Design review of the part built by this model. Coordinates are the model's own, in mm. Face numbers are marked on the shaded views. Give positions to 0.01 mm unless a question says otherwise; leave off trailing zeros. Order: outer loops, then holes, each group sorted by start corner. A loop starts at its lowest first (then second) coordinate and runs counter-clockwise, first axis right, second up. Notation, with made-up numbers: (59.5, 19.5) -> (86.5, 19.5) arc R27 ccw to (86.5, 36.5) -> close; hole circle Ø10 at (-19.5, 1). An arc over 180 degrees is marked (long way). Use a Markdown table: item, result. Add a question column.
```python
from build123d import *

# Parameters (mm, degrees)
BOSS_EXTRUDE1_DEPTH = 0.508
SKETCH2_R           = 7.874
SKETCH2_R_2         = 6.35
CUT_EXTRUDE2_DEPTH  = 0.254
SKETCH5_R           = 6.354160617
CUT_EXTRUDE3_DEPTH  = 68.821805137
SKETCH6_R           = 5.461
CUT_EXTRUDE4_DEPTH  = 68.821805137
SKETCH7_W           = 19.558
SKETCH7_H           = 1.016
CUT_EXTRUDE5_DEPTH  = 68.823232008
SKETCH8_W           = 6.35
SKETCH8_H           = 0.254
BOSS_EXTRUDE2_DEPTH = 2.032
SKETCH10_W          = 11.303182767
SKETCH10_H          = 0.254
BOSS_EXTRUDE3_DEPTH = 2.032
SKETCH11_W          = 6.35
SKETCH11_H          = 0.254
BOSS_EXTRUDE4_DEPTH = 2.032
SKETCH12_W          = 11.938
SKETCH12_H          = 0.254
BOSS_EXTRUDE5_DEPTH = 2.032


with BuildPart() as part:
    # Sketch1 → Boss-Extrude1 (new body)
    with BuildSketch(Plane.XY):
        with BuildLine():
            ThreePointArc((0, -10.16), (10.16, 0), (0, 10.16))
            Line((0, 10.16), (-67.056, 10.16))
            Line((-67.056, 10.16), (-67.056, -10.16))
            Line((-67.056, -10.16), (0, -10.16))
        make_face()
    extrude(amount=BOSS_EXTRUDE1_DEPTH)

    # Sketch2 → Cut-Extrude2 (cut)
    with BuildSketch(Plane.XY.offset(0.508)):
        with Locations((-54.61, 0)):
            Circle(SKETCH2_R)
        with Locations((-35.814, 0)):
            Circle(SKETCH2_R_2)
    extrude(amount=-CUT_EXTRUDE2_DEPTH, mode=Mode.SUBTRACT)

    # Sketch5 → Cut-Extrude3 (cut, through all)
    with BuildSketch(Plane.XY.offset(0.254)):
        with Locations((-35.814, 0)):
            Circle(SKETCH5_R)
    extrude(amount=-CUT_EXTRUDE3_DEPTH, mode=Mode.SUBTRACT)

    # Sketch6 → Cut-Extrude4 (cut, through all)
    with BuildSketch(Plane.XY.offset(0.254)):
        with Locations((-54.61, 0)):
            Circle(SKETCH6_R)
    extrude(amount=-CUT_EXTRUDE4_DEPTH, mode=Mode.SUBTRACT)

    # Sketch7 → Cut-Extrude5 (cut, through all)
    with BuildSketch(Plane(origin=(0, 0, 0), x_dir=(-1, 0, 0), z_dir=(0, 0, -1))):
        with Locations((50.927, 9.652)):
            Rectangle(SKETCH7_W, SKETCH7_H)
        with Locations((50.927, -9.652)):
            Rectangle(SKETCH7_W, SKETCH7_H)
    extrude(amount=-CUT_EXTRUDE5_DEPTH, mode=Mode.SUBTRACT)

    # Sketch8 → Boss-Extrude2 (add)
    with BuildSketch(Plane(origin=(0, 0, 0), x_dir=(-1, 0, 0), z_dir=(0, 0, -1))):
        with Locations((63.881, 10.033)):
            Rectangle(SKETCH8_W, SKETCH8_H)
    extrude(amount=BOSS_EXTRUDE2_DEPTH)

    # Sketch10 → Boss-Extrude3 (add)
    with BuildSketch(Plane(origin=(0, 0, 0), x_dir=(-1, 0, 0), z_dir=(0, 0, -1))):
        with Locations((35.496408617, 10.033)):
            Rectangle(SKETCH10_W, SKETCH10_H)
    extrude(amount=BOSS_EXTRUDE3_DEPTH)

    # Sketch11 → Boss-Extrude4 (add)
    with BuildSketch(Plane(origin=(0, 0, 0), x_dir=(-1, 0, 0), z_dir=(0, 0, -1))):
        with Locations((63.881, -10.033)):
            Rectangle(SKETCH11_W, SKETCH11_H)
    extrude(amount=BOSS_EXTRUDE4_DEPTH)

    # Sketch12 → Boss-Extrude5 (add)
    with BuildSketch(Plane(origin=(0, 0, 0), x_dir=(-1, 0, 0), z_dir=(0, 0, -1))):
        with Locations((35.179, -10.033)):
            Rectangle(SKETCH12_W, SKETCH12_H)
    extrude(amount=BOSS_EXTRUDE5_DEPTH)


solid = part.part
```
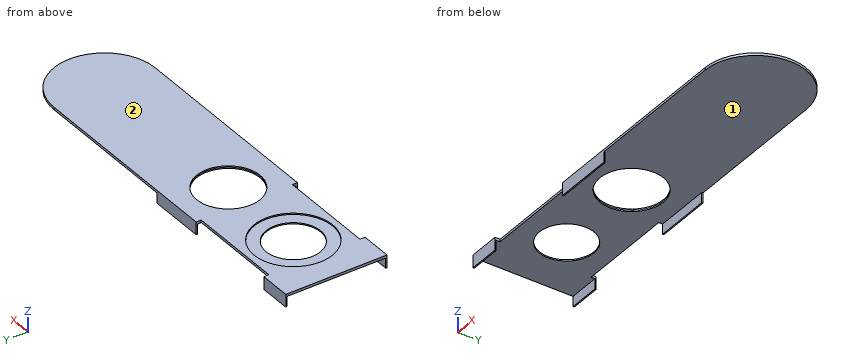
1) Add section B-B (z = -1.35). Give the boundary of the cut face in (x, y).
2) Add section A-A (y = 0). Give the number of separate pieces and of enclosed holes in the cut face, then the cut area to 3 significant figures.
3) For L1, parallel to Y at x = -54.61, z = 0.2; L2, parallel to Y at x = -35.5, z = -1.7; L3, parallel to Z at x = -13.5, y = -7.5, list the stretches that pass through material, from the lowest coordinate up. Write a range as [from, to].
4) Insertion check: pin 1 (11.5 mm diameter, centred on x = -35.814, y = 0, fed in from +Z); pin 2 (0.5 mm diameter, centred on y = -10, z = -0.5, fed in from +X); pin 3 (1.5 mm diameter, centred on x = -16, y = -6.5, fed in from -Z); pin 4 (8 mm diameter, centred on x = -56, y = -3, fed in from +Z). Each pin has a flat end and moves straight along its axis. Give the tip position at first contact, or say it passes through.
5) Add section D-D (x = -44.5). Give the boundary of the cut face in (y, z).
6) Add section C-C (x = -54.61). Give the boundary of the cut face in (y, z).
7) The part is to be moulded in two halves that separate along Y. For the marked faces 1 and 2, say which applies: +Y half, -Y half, draft (parallel to the pull), parting line (faces both ways), or undercut.
Worked answers:
| question | item | result |
|---|---|---|
| 1 | outline | (-67.06, -10.16) -> (-60.71, -10.16) -> (-60.71, -9.91) -> (-67.06, -9.91) -> close; (-67.06, 9.91) -> (-60.71, 9.91) -> (-60.71, 10.16) -> (-67.06, 10.16) -> close; (-41.15, -10.16) -> (-29.21, -10.16) -> (-29.21, -9.91) -> (-41.15, -9.91) -> close; (-41.15, 9.91) -> (-29.84, 9.91) -> (-29.84, 10.16) -> (-41.15, 10.16) -> close |
| 2 | separate pieces | 3 |
| 2 | enclosed holes | 0 |
| 2 | area | 26.0 mm^2 |
| 3 | L1 | [-9.14, -5.46], [5.46, 9.14] |
| 3 | L2 | [-10.16, -9.91], [9.91, 10.16] |
| 3 | L3 | [0, 0.51] |
| 4 | pin 1 | through |
| 4 | pin 2 | x = -29.21 |
| 4 | pin 3 | z = 0 |
| 4 | pin 4 | z = 0.25 |
| 5 | outline | (-9.14, 0) -> (9.14, 0) -> (9.14, 0.51) -> (-9.14, 0.51) -> close |
| 6 | outline | (-9.14, 0) -> (-5.46, 0) -> (-5.46, 0.25) -> (-7.87, 0.25) -> (-7.87, 0.51) -> (-9.14, 0.51) -> close; (5.46, 0) -> (9.14, 0) -> (9.14, 0.51) -> (7.87, 0.51) -> (7.87, 0.25) -> (5.46, 0.25) -> close |
| 7 | face 1 | undercut |
| 7 | face 2 | draft |
